The listing builds one solid part. Answer for the finished solid, in the listing's coordinates (mm). Face numbers are marked on the shaded views. A direction names the side the tool comes from. Give positions to 0.01 mm unless a question says otherwise; leave off trailing zeros. Write each loop counter-clockwise with the first axis right and the second up, starting at its lowest first coordinate (ties: lowest second). Pieces come first, ordered by that corner, then holes. Notation, with made-up numbers: (9, 20) -> (55, 20) arc R11 ccw to (55, 24) -> close; hole circle Ø11 at (4, 71.25). An arc over 180 degrees is marked (long way). Put each result on its own line as item: value. Start each with the question number.
1) A cutting plane is placed at A-A (z = 7.5). Write down the section's boundary in (x, y).
2) Find the intervals of material crossed by line 1 along Z through (x, y) = (-15, -0.75); line 2 along Y through (x, z) = (-44, 10.25), in increasing order. Write a range as from..to.
3) A cutting plane is placed at B-B (x = -40). Write down the section's boundary in (y, z), then the cut area to 3 significant figures.
4) A cutting plane is placed at D-D (z = 4). Write down the section's boundary in (x, y).
5) Flat-ended cylindrical pins translate along their axes: pin 1 Ø2.5 at (y, z) = (-40, 7.5) entering from +X; pin 2 Ø7.5 at (x, z) = (-23, 6) entering from -Y; pin 3 Ø7.5 at (y, z) = (-37, 10.5) entering from -X. Find the tip coordinate at first contact, or state that the pin passes through.
6) For the marked faces 1 and 2, determine the directions among +Z, -Z, +X, -X, +Y, -Y from which every point of the face is accessible in a straight line to the end or side of a thin tool.
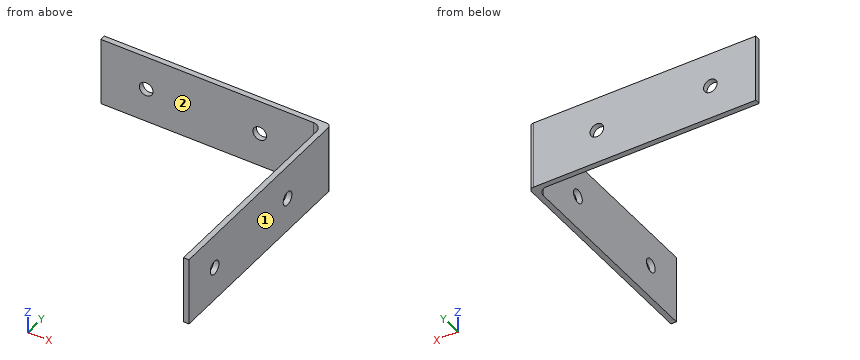
from build123d import *

# Parameters (mm, degrees)
PAD_DEPTH       = 15
SKETCH001_R     = 1.5
POCKET_DEPTH    = 1.201
SKETCH002_R     = 1.5
POCKET001_DEPTH = 1.201
FILLET_R        = 2
FILLET001_R     = 1


with BuildPart() as part:
    # Sketch → Pad (new body)
    with BuildSketch(Plane.XY):
        Polygon((-50, 0), (0, 0), (0, -48.8), (-1.2, -48.8), (-1.2, -1.2), (-50, -1.2), align=None)
    extrude(amount=PAD_DEPTH)

    # Sketch001 (on Face5 of Pad) → Pocket (cut, through all)
    with BuildSketch(Plane.XZ.offset(1.2)):
        with Locations((-40, 7.5)):
            Circle(SKETCH001_R)
        with Locations((-15, 7.5)):
            Circle(SKETCH001_R)
    extrude(amount=-POCKET_DEPTH, mode=Mode.SUBTRACT)

    # Sketch002 (on Face10 of Pocket) → Pocket001 (cut, through all)
    with BuildSketch(Plane(origin=(-1.2, 0, 0), x_dir=(0, -1, 0), z_dir=(-1, 0, 0))):
        with Locations((15, 7.5)):
            Circle(SKETCH002_R)
        with Locations((40, 7.5)):
            Circle(SKETCH002_R)
    extrude(amount=-POCKET001_DEPTH, mode=Mode.SUBTRACT)

    # Fillet
    fillet_edges = [part.edges().sort_by_distance(p)[0] for p in [
        (-1.2, -1.2, 7.5),
    ]]
    fillet(fillet_edges, radius=FILLET_R)

    # Fillet001
    fillet001_edges = [part.edges().sort_by_distance(p)[0] for p in [
        (0, 0, 7.5),
    ]]
    fillet(fillet001_edges, radius=FILLET001_R)


solid = part.part
Reply:
1. outline: (-50, -1.2) -> (-41.5, -1.2) -> (-41.5, 0) -> (-50, 0) -> close; (-38.5, -1.2) -> (-16.5, -1.2) -> (-16.5, 0) -> (-38.5, 0) -> close; (-13.5, -1.2) -> (-3.2, -1.2) arc R2 cw to (-1.2, -3.2) -> (-1.2, -13.5) -> (0, -13.5) -> (0, -1) arc R1 ccw to (-1, 0) -> (-13.5, 0) -> close; (-1.2, -48.8) -> (0, -48.8) -> (0, -41.5) -> (-1.2, -41.5) -> close; (-1.2, -38.5) -> (0, -38.5) -> (0, -16.5) -> (-1.2, -16.5) -> close
2. line 1: z = 0..6, 9..15
2. line 2: y = -1.2..0
3. outline: (-1.2, 0) -> (0, 0) -> (0, 6) -> (-1.2, 6) -> close; (-1.2, 9) -> (0, 9) -> (0, 15) -> (-1.2, 15) -> close
3. area: 14.4 mm2
4. outline: (-50, -1.2) -> (-3.2, -1.2) arc R2 cw to (-1.2, -3.2) -> (-1.2, -48.8) -> (0, -48.8) -> (0, -1) arc R1 ccw to (-1, 0) -> (-50, 0) -> close
5. pin 1: passes through
5. pin 2: stops at y = -1.2
5. pin 3: stops at x = -1.2
6. face 1: +Z, -Z, +X, +Y, -Y
6. face 2: +Z, -Z, -X, -Y
